from build123d import *

# Parameters (mm, degrees)
SKETCH1_R           = 71.12
BOSS_EXTRUDE1_DEPTH = 7.62
FILLET1_R           = 0.9906
SKETCH3_R           = 6.35
BOSS_EXTRUDE2_DEPTH = 7.62
SKETCH5_R           = 6.35
CUT_EXTRUDE1_DEPTH  = 233.857192717


with BuildPart() as part:
    # Sketch1 → Boss-Extrude1 (new body)
    with BuildSketch(Plane(origin=(0, 0, 0), x_dir=(1, 0, 0), z_dir=(0, 1, 0))):
        with Locations(Location((0, 0, 0), (0, 0, 270))):
            Circle(SKETCH1_R)
    extrude(amount=BOSS_EXTRUDE1_DEPTH)

    # Fillet1
    fillet1_edges = [part.edges().sort_by_distance(p)[0] for p in [
        (0, 0, -71.12),
        (0, 7.62, -71.12),
    ]]
    fillet(fillet1_edges, radius=FILLET1_R)

    # Sketch3 → Boss-Extrude2 (add)
    with BuildSketch(Plane.XY.offset(45.72)):
        with BuildLine():
            Line((0, 0), (43.18, 0))
            Line((43.18, 0), (-61.579637217, -167.864725032))
            ThreePointArc((-61.579637217, -167.864725032), (-100.613254195, -177.896447691), (-112.513352174, -139.391300217))
            Line((-112.513352174, -139.391300217), (-43.18, 0))
            Line((-43.18, 0), (0, 0))
        make_face()
        with Locations((-86.36, -152.4)):
            Circle(SKETCH3_R, mode=Mode.SUBTRACT)
    boss_extrude2 = extrude(amount=BOSS_EXTRUDE2_DEPTH)

    # Mirror1: Boss-Extrude2 across plane
    add(boss_extrude2.mirror(Plane.XY))

    # Sketch5 → Cut-Extrude1 (cut, through all)
    with BuildSketch(Plane(origin=(0, 7.62, 0), x_dir=(1, 0, 0), z_dir=(0, 1, 0))):
        with Locations(Location((0, 0, 0), (0, 0, 270))):
            Circle(SKETCH5_R)
    extrude(amount=-CUT_EXTRUDE1_DEPTH, mode=Mode.SUBTRACT)


solid = part.part
Work out the finished part from the listing and answer in its coordinate system (mm). A direction names the side the tool comes from. Give positions to 0.01 mm unless a question says otherwise; leave off trailing zeros. Write each loop counter-clockwise with the first axis right and the second up, starting at its lowest first coordinate (ties: lowest second). Pieces come first, ordered by that corner, then holes. Notation, with made-up numbers: (15.5, -15.5) - (31.5, -15.5) arc R21 cw to (31.5, 11.5) - close; hole circle Ø1 at (-26, -40). An arc over 180 degrees is marked (long way). One line per item, written item: value. Start each with the question number.
1. For a pull along X with two mould halves and no side action, classify faces 1 (the cylindrical face through (-69.43, 3.77, -15.42)), 2 (the cylindrical face through (-83.43, -158.034, 49.477)), 3 (the cylindrical face through (-83.43, -158.034, -49.477)), 4 (the flat face through (-53, -90, -45.72)) as +X half, -X half, draft (parallel to the pull), parting line (faces both ways), or undercut.
2. Find section A-A (z = 0). Write down the section's boundary in (x, y), then the cut area to 3 significant figures.
3. Find section C-C (x = -77.5). Write down the section's boundary in (y, z).
4. Find section B-B (y = -29.5). Write down the section's boundary in (x, z), then the cut area to 3 significant figures.
5. Consider probe 1 along Z at (x, y) = (2.5, -16.5); probe 2 along Y at (x, z) = (-86.36, 49.75); probe 3 along Y at (x, z) = (-86, 50). Determine where each line is inside the solid, lowest interval first.
6. Given pin 1 (11.5 mm diameter, centred on x = 0, z = 0, fed in from +Y); pin 2 (10 mm diameter, centred on x = -56, y = -47, fed in from +Z); pin 3 (8 mm diameter, centred on x = -34, z = -46, fed in from -Y); pin 4 (8 mm diameter, centred on x = -41.5, z = -44, fed in from -Y), each flat-ended and moving along its own axis, determine where each tip first touches the part or whether it passes through.
7. Find section D-D (y = -152.4). Write down the section's boundary in (x, z).
8. For faces 5 (the flat face through (-8.47, -82.76, 49.48)), 6 (the cylindrical face through (-3.86, 3.86, -5.04)), 7 (the flat face through (-53, -90, -53.34)), 8 (the flat face through (-53, -90, 45.72)), 9 (the flat face through (-53, -90, 53.34)), determine the directions among +Z, -Z, +X, -X, +Y, -Y from which every point of the face is accessible in a straight line to the end or side of a thin tool.
Geometry results:
1. face 1: parting line
1. face 2: undercut
1. face 3: undercut
1. face 4: draft
2. outline: (-71.12, 0.99) arc R0.99 ccw to (-70.13, 0) - (-6.35, 0) - (-6.35, 7.62) - (-70.13, 7.62) arc R0.99 ccw to (-71.12, 6.63) - close; (6.35, 0) - (70.13, 0) arc R0.99 ccw to (71.12, 0.99) - (71.12, 6.63) arc R0.99 ccw to (70.13, 7.62) - (6.35, 7.62) - close
2. area: 986 mm2
3. outline: (-180.23, -53.34) - (-69, -53.34) - (-69, -45.72) - (-180.23, -45.72) - close; (-180.23, 45.72) - (-69, 45.72) - (-69, 53.34) - (-180.23, 53.34) - close
4. outline: (-57.85, -53.34) - (24.77, -53.34) - (24.77, -45.72) - (-57.85, -45.72) - close; (-57.85, 45.72) - (24.77, 45.72) - (24.77, 53.34) - (-57.85, 53.34) - close
4. area: 1,260 mm2
5. probe 1: -53.34 to -45.72, 45.72 to 53.34
5. probe 2: -181.61 to -158.75, -146.05 to -86.81
5. probe 3: -181.61 to -158.74, -146.06 to -86.09
6. pin 1: through
6. pin 2: z = 53.34
6. pin 3: y = -130.08
6. pin 4: y = -141.48
7. outline: (-115.57, -53.34) - (-92.71, -53.34) - (-92.71, -45.72) - (-115.57, -45.72) - close; (-115.57, 45.72) - (-92.71, 45.72) - (-92.71, 53.34) - (-115.57, 53.34) - close; (-80.01, -53.34) - (-51.93, -53.34) - (-51.93, -45.72) - (-80.01, -45.72) - close; (-80.01, 45.72) - (-51.93, 45.72) - (-51.93, 53.34) - (-80.01, 53.34) - close
8. face 5: +Z, -Z, +X, -Y
8. face 6: +Y, -Y
8. face 7: -Z, +X, -X, -Y
8. face 8: +X, -X, -Y
8. face 9: +Z, +X, -X, -Y
